Check sheet for the modelled part. Datum: model origin and axes. Units: mm. Face numbers are marked on the shaded views. Give positions to 0.01 mm unless a question says otherwise; leave off trailing zeros. Loops run counter-clockwise (first coordinate to the right, second up) from the corner with the lowest first, then second, coordinate; pieces in that order, holes last. Notation, with made-up numbers: (48.5, -9.75) - (74.5, -9.75) arc R31 ccw to (74.5, 19.25) - close; hole circle Ø4 at (-11, 78.25). An arc over 180 degrees is marked (long way). Answer in a Markdown table with one row per item. Add a question column.
(1) Draft check along Y on the marked faces 1, 2 and 3. Enter one of: released by +Y, released by -Y, zero draft, split by the parting line, or undercut.
(2) Thickness scan on L1, parallel to Y at x = 0.75, z = 1.4; L2, parallel to Z at x = -0.05, y = -3.75; L3, parallel to Y at x = 0.05, z = 0.05. Record the ranges inside material, lowest first.
(3) Sectioned sample at A-A on y = -2.5. Enter the section's corners in (x, z), then the cut area to 3 significant figures.
(4) Go/stop test with a flat-tipped pin: P1, Ø1.5, axis at x = 0, y = -2.5, coming from the -Z side. Record where the tip stops, or that it passes through.
from build123d import *

# Parameters (mm, degrees)
SKETCH2_R           = 0.225118876
BOSS_EXTRUDE1_DEPTH = 10


with BuildPart() as part:
    # Sketch1 → Revolve1 (revolve)
    with BuildSketch(Plane.XY, mode=Mode.PRIVATE) as revolve1_sk:
        with BuildLine():
            Line((0, 0), (0, 6.422564509))
            ThreePointArc((0, 6.422564509), (1.15329097, 5.759594151), (1.5, 4.47530345))
            Line((1.5, 4.47530345), (1.5, 1.47530345))
            Line((1.5, 1.47530345), (1.87, 1.47530345))
            Line((1.87, 1.47530345), (1.87, 0))
            Line((1.87, 0), (0, 0))
        make_face()
    revolve(revolve1_sk.sketch.rotate(Axis((0, 0, 0), (0, 1, 0)), 90), axis=Axis((0, 0, 0), (0, 1, 0)))

    # Sketch2 → Boss-Extrude1 (add)
    with BuildSketch(Plane(origin=(0, 0, 0), x_dir=(-1, 0, 0), z_dir=(0, -1, 0))):
        with Locations(Location((0, 0.822285039, 0), (0, 0, 90))):
            Circle(SKETCH2_R)
        with Locations(Location((0, -0.822285039, 0), (0, 0, 270))):
            Circle(SKETCH2_R)
    extrude(amount=BOSS_EXTRUDE1_DEPTH)


solid = part.part
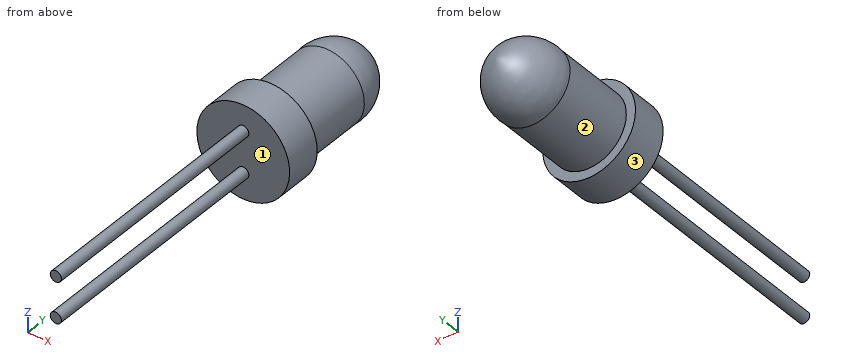
Reply:
| question | item | result |
|---|---|---|
| 1 | face 1 | released by -Y |
| 1 | face 2 | undercut |
| 1 | face 3 | zero draft |
| 2 | L1 | 0 to 1.48 |
| 2 | L2 | -1.04 to -0.6, 0.6 to 1.04 |
| 2 | L3 | 0 to 6.41 |
| 3 | outline | circle Ø0.45 at (0, -0.82); circle Ø0.45 at (0, 0.82) |
| 3 | area | 0.318 mm^2 |
| 4 | P1 | z = -1.05 |
